Model file for the job. Use its own axes, mm. A direction names the side the tool comes from. Give positions to 0.01 mm unless a question says otherwise; leave off trailing zeros. Write each loop counter-clockwise with the first axis right and the second up, starting at its lowest first coordinate (ties: lowest second). Pieces come first, ordered by that corner, then holes. Notation, with made-up numbers: M -29,-11 L 25,-11 A38 cw 25,27 Z; hole C 74,16.25 d8. An arc over 180 degrees is marked long. Answer as a JSON object with one key per item and string values. Group by question number.
```python
from build123d import *

# Parameters (mm, degrees)
SKETCH1_W           = 346.7
SKETCH1_H           = 376.55000001
BOSS_EXTRUDE1_DEPTH = 18
SKETCH2_W           = 346.7
SKETCH2_H           = 18
CUT_EXTRUDE1_DEPTH  = 6.35
FILLET1_R           = 9.525
SKETCH3_W           = 346.7
SKETCH3_H           = 19.05
CUT_EXTRUDE2_DEPTH  = 6.35
SKETCH4_W           = 346.7
SKETCH4_H           = 12.7
CUT_EXTRUDE3_DEPTH  = 19
FILLET2_R           = 9.525


with BuildPart() as part:
    # Sketch1 → Boss-Extrude1 (new body)
    with BuildSketch(Plane(origin=(0, 0, 0), x_dir=(1, 0, 0), z_dir=(0, 1, 0))):
        with Locations((173.35, -188.275000005)):
            Rectangle(SKETCH1_W, SKETCH1_H)
    extrude(amount=BOSS_EXTRUDE1_DEPTH)

    # Sketch2 → Cut-Extrude1 (cut)
    with BuildSketch(Plane(origin=(0, 18, 0), x_dir=(1, 0, 0), z_dir=(0, 1, 0))):
        with Locations((173.35, -329.45000001)):
            Rectangle(SKETCH2_W, SKETCH2_H)
    extrude(amount=-CUT_EXTRUDE1_DEPTH, mode=Mode.SUBTRACT)

    # Fillet1
    fillet1_edges = [part.edges().sort_by_distance(p)[0] for p in [
        (173.35, 0, 376.55000001),
    ]]
    fillet(fillet1_edges, radius=FILLET1_R)

    # Sketch3 → Cut-Extrude2 (cut)
    with BuildSketch(Plane(origin=(0, 18, 0), x_dir=(1, 0, 0), z_dir=(0, 1, 0))):
        with Locations((173.35, -9.525)):
            Rectangle(SKETCH3_W, SKETCH3_H)
    extrude(amount=-CUT_EXTRUDE2_DEPTH, mode=Mode.SUBTRACT)

    # Sketch4 → Cut-Extrude3 (cut, through all)
    with BuildSketch(Plane(origin=(0, 18, 0), x_dir=(1, 0, 0), z_dir=(0, 1, 0))):
        with Locations((173.35, -370.20000001)):
            Rectangle(SKETCH4_W, SKETCH4_H)
    extrude(amount=-CUT_EXTRUDE3_DEPTH, mode=Mode.SUBTRACT)

    # Fillet2
    fillet2_edges = [part.edges().sort_by_distance(p)[0] for p in [
        (173.35, 0, 363.85000001),
    ]]
    fillet(fillet2_edges, radius=FILLET2_R)


solid = part.part
```
Q1. Wall check: L1, parallel to Z at x = 242, y = 14; L2, parallel to Z at x = 317.5, y = 8.5; L3, parallel to Z at x = 156, y = 7.25. Give the ranges that are in metal, low to high.
Q2. 3-axis set-ups, long thin cutter, end or side, ignore diameter. For faces 1 (the flat face through (171, 11.65, 9)), 2 (the cylindrical face through (175.78, 2.72, 360.99)): which of +Z, -Z, +X, -X, +Y, -Y reach the whole face in a straight line?
Q3. Two-plate mould, pull along Z, no slides. Class faces 3 (the flat face through (171, 14, 363.85)), 4 (the flat face through (171, 11.65, 329)), 5 (the flat face through (346.7, 9, 184)): +Z half, -Z half, draft (parallel to the pull), parting line (faces both ways), or undercut.
Q4. Slice it at A-A, the plane x = 296.5. Write the cut outline in (y, z) (3 decimals).
Q5. Drop flat-ended pins along their axis: P1, Ø3, axis at x = 94.5, y = 14, coming from the -Z side; P2, Ø21, axis at x = 178, z = 8.5, coming from the +Y side. Give the stop position or say it passes through.
Q6. Slice it at B-B, the plane z = 325. Write the cut outline in (x, y).
Solved:
{
 "1": {"L1": "z = 19.05 to 320.45, 338.45 to 363.85", "L2": "z = 0 to 363.79", "L3": "z = 0 to 363.57"},
 "2": {"face 1": "-Z, +X, -X, +Y", "face 2": "+Z, +X, -X, -Y"},
 "3": {"face 3": "+Z half", "face 4": "undercut", "face 5": "draft"},
 "4": {"outline": "M 0,0 L 11.65,0 L 11.65,19.05 L 18,19.05 L 18,320.45 L 11.65,320.45 L 11.65,338.45 L 18,338.45 L 18,363.85 L 9.525,363.85 A9.525 ccw 0,354.325 Z"},
 "5": {"P1": "stops at z = 19.05", "P2": "stops at y = 11.65"},
 "6": {"outline": "M 0,0 L 346.7,0 L 346.7,11.65 L 0,11.65 Z"}
}
